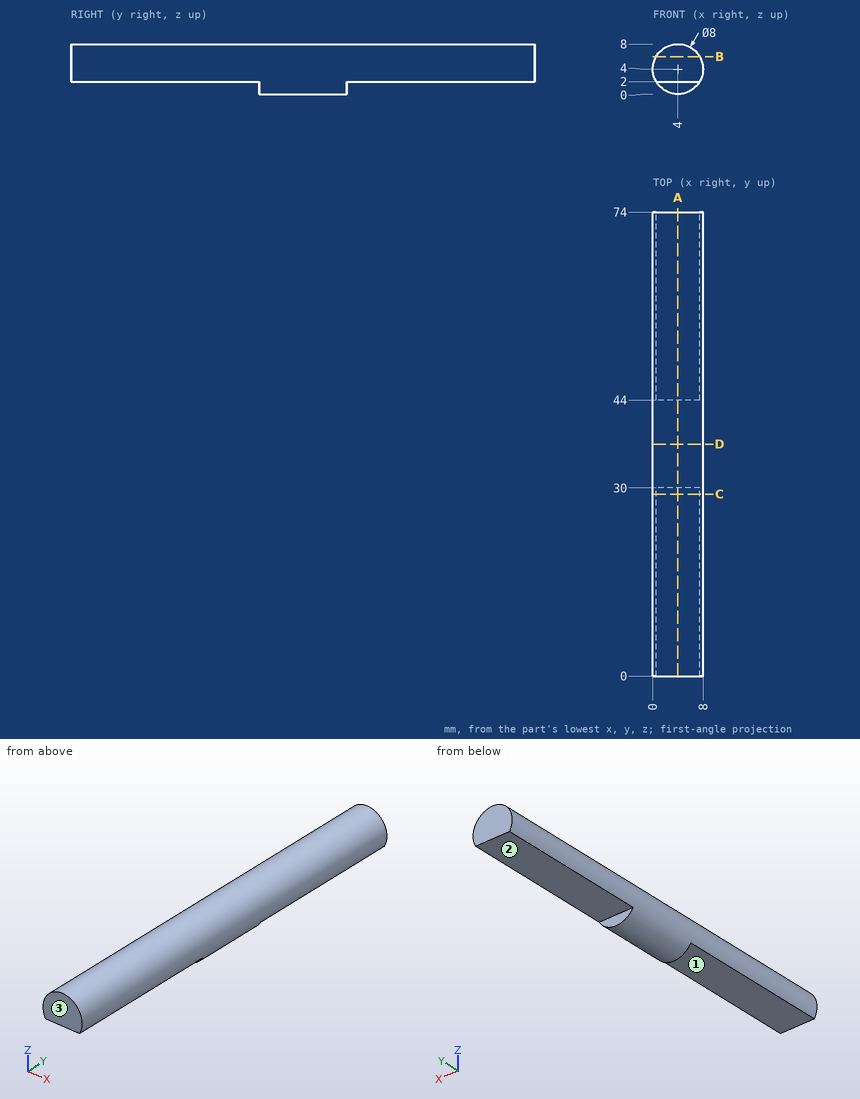
Job drawing, mm, ordinate dimensions from the low corner. One solid piece. A direction names the side the tool comes from. Give positions to 0.01 mm unless a question says otherwise; leave off trailing zeros. Loops run counter-clockwise (first coordinate to the right, second up) from the corner with the lowest first, then second, coordinate; pieces in that order, holes last. Notation, with made-up numbers: M 22.5,67.25 L 31.5,67.25 A17 ccw 31.5,91.25 Z; hole C 89,-12 d10. An arc over 180 degrees is marked long. Answer in a Markdown table with one row per item. Add a question column.
Item 1: Band-saw the part on C-C on y = 29. Give the cut face in (x, z), then the cut area to 3 significant figures.
Item 2: Tool access for the marked faces 1, 2 and 3: list every direction of +Z, -Z, +X, -X, +Y, -Y with a clear straight run to the whole face (end or side of a thin tool).
Item 3: Band-saw the part on D-D on y = 37. Give the cut face in (x, z), then the cut area to 3 significant figures.
Item 4: Band-saw the part on A-A on x = 4. Give the cut face in (y, z), then the cut area to 3 significant figures.
Item 5: Band-saw the part on B-B on z = 6. Give the cut face in (x, y).
Item 6: Probe probe 1 along Y at (x, z) = (1, 1.75); probe 2 along Z at (x, y) = (3.5, 13.5); probe 3 along Z at (x, y) = (3, 34). List the from-to ranges inside material, lowest first.
Item 7: Drop flat-ended pins along their axis: P1, Ø3, axis at x = 6, y = 32, coming from the +Z side; P2, Ø3.5, axis at x = 4, y = 62, coming from the -Z side; P3, Ø2, axis at y = 30, z = 1, coming from the +X side. Give the stop position or say it passes through.
Reply:
| question | item | result |
|---|---|---|
| 1 | outline | M 0.54,2 L 7.46,2 A4 ccw long Z |
| 1 | area | 40.4 mm^2 |
| 2 | face 1 | -Z, +X, -X, -Y |
| 2 | face 2 | -Z, +X, -X, +Y |
| 2 | face 3 | +Z, -Z, +X, -X, -Y |
| 3 | outline | C 4,4 d8 |
| 3 | area | 50.3 mm^2 |
| 4 | outline | M 0,2 L 30,2 L 30,0 L 44,0 L 44,2 L 74,2 L 74,8 L 0,8 Z |
| 4 | area | 472 mm^2 |
| 5 | outline | M 0.54,0 L 7.46,0 L 7.46,74 L 0.54,74 Z |
| 6 | probe 1 | y = 30 to 44 |
| 6 | probe 2 | z = 2 to 7.97 |
| 6 | probe 3 | z = 0.13 to 7.87 |
| 7 | P1 | stops at z = 7.97 |
| 7 | P2 | stops at z = 2 |
| 7 | P3 | stops at x = 7.46 |
